Here's how the part is built. I have some questions about the finished solid (model axes, mm). Face numbers are marked on the shaded views. A direction names the side the tool comes from. Round coordinates to 2 decimals unless told otherwise and drop trailing zeros. Order: outer loops, then holes, each group sorted by start corner. A loop starts at its lowest first (then second) coordinate and runs counter-clockwise, first axis right, second up.
```python
from build123d import *

# Parameters (mm, degrees)
SKETCH2_W             = 5.91625
SKETCH2_H             = 9
BOSS_EXTRUDE1_DEPTH   = 2
SKETCH2_W_2           = 9.732
SKETCH2_H_2           = 9.5
BOSS_EXTRUDE1_2_DEPTH = 2
BOSS_EXTRUDE1_3_DEPTH = 2
SKETCH3_W             = 2
SKETCH3_H             = 1
BOSS_EXTRUDE2_DEPTH   = 13
FILLET1_R             = 4
CUT_EXTRUDE1_DEPTH    = 83.031058661
M3_CLEARANCE_HOLE2_D  = 3.6


with BuildPart() as part:
    # Sketch2 → Boss-Extrude1 (new body)
    with BuildSketch(Plane.XY.offset(11.211435671)):
        with Locations((2.267401673, -43.012787822)):
            Rectangle(SKETCH2_W, SKETCH2_H)
    extrude(amount=BOSS_EXTRUDE1_DEPTH)



with BuildPart() as body_2:
    # Sketch2 → Boss-Extrude1 2 (new body)
    with BuildSketch(Plane.XY.offset(11.211435671)):
        with Locations((0.359526673, -72.762787822)):
            Rectangle(SKETCH2_W_2, SKETCH2_H_2)
    extrude(amount=BOSS_EXTRUDE1_2_DEPTH)


with BuildPart() as body_3:
    # Sketch2 → Boss-Extrude1 3 (new body)
    with BuildSketch(Plane.XY.offset(11.211435671)):
        with Locations((0.359526673, -13.262787822)):
            Rectangle(SKETCH2_W_2, SKETCH2_H_2)
    extrude(amount=BOSS_EXTRUDE1_3_DEPTH)


with BuildPart() as part_1:
    add(part.part)

    add(body_2.part)  # Boss-Extrude2 merges body 2

    add(body_3.part)  # Boss-Extrude2 merges body 3
    # Sketch3 → Boss-Extrude2 (add)
    with BuildSketch(Plane.XY.offset(13.211435671)):
        Polygon((-0.690723327, -17.012787822), (-0.690723327, -38.512787822), (-0.690723327, -47.512787822), (-0.690723327, -68.012787822), (1.309276673, -68.012787822), (1.309276673, -17.012787822), align=None)
        with Locations((0.309276673, -68.512787822)):
            Rectangle(SKETCH3_W, SKETCH3_H)
    extrude(amount=BOSS_EXTRUDE2_DEPTH)

    # Fillet1
    # the kernel refuses this fillet: 4 mm, written as the material it adds along each edge
    with BuildSketch(Plane(origin=(-0.690723327, -17.012787822, 13.211435671), x_dir=(0, 0, 1), z_dir=(0, -1, 0)), Plane(origin=(-0.690723327, -68.012787822, 13.211435671), x_dir=(0, 0, 1), z_dir=(0, -1, 0))) as fillet1_piece_1:
        with BuildLine():
            CenterArc((3.995754239, 4), FILLET1_R, 182.64012102, 87.35987898)
            Line((0, 3.81575), (0, 0))
            Line((0, 0), (3.995754239, 0))
        make_face()
    extrude(amount=1)
    with BuildSketch(Plane(origin=(1.309276673, -17.012787822, 13.211435671), x_dir=(0, 1, 0), z_dir=(-1, 0, 0))) as fillet1_piece_2:
        with BuildLine():
            CenterArc((FILLET1_R, -FILLET1_R), FILLET1_R, 90, 90)
            Line((0, -FILLET1_R), (0, 0))
            Line((0, 0), (FILLET1_R, 0))
        make_face()
    extrude(amount=2)
    with BuildSketch(Plane(origin=(1.309276673, -17.012787822, 13.211435671), x_dir=(1, 0, 0), z_dir=(0, -1, 0))) as fillet1_piece_3_section:
        with BuildLine():
            CenterArc((FILLET1_R, FILLET1_R), FILLET1_R, 180, 90)
            Line((0, FILLET1_R), (0, 0))
            Line((0, 0), (FILLET1_R, 0))
        make_face()
    fillet1_piece_3 = extrude(amount=1, mode=Mode.PRIVATE)
    fillet1_piece_3 = split(fillet1_piece_3, bisect_by=Plane(origin=(5.225526673, -17.012787822, 13.211435671), z_dir=(-1, 0, 0)), keep=Keep.TOP, mode=Mode.PRIVATE)
    add(fillet1_piece_3)
    with BuildSketch(Plane(origin=(1.309276673, -38.512787822, 13.211435671), x_dir=(1, 0, 0), z_dir=(0, -1, 0))) as fillet1_piece_4_section:
        with BuildLine():
            CenterArc((FILLET1_R, FILLET1_R), FILLET1_R, 180, 90)
            Line((0, FILLET1_R), (0, 0))
            Line((0, 0), (FILLET1_R, 0))
        make_face()
    fillet1_piece_4 = extrude(amount=9, mode=Mode.PRIVATE)
    fillet1_piece_4 = split(fillet1_piece_4, bisect_by=Plane(origin=(5.225526673, -38.512787822, 13.211435671), z_dir=(-1, 0, 0)), keep=Keep.TOP, mode=Mode.PRIVATE)
    add(fillet1_piece_4)
    with BuildSketch(Plane(origin=(1.309276673, -68.012787822, 13.211435671), x_dir=(1, 0, 0), z_dir=(0, -1, 0))) as fillet1_piece_5_section:
        with BuildLine():
            CenterArc((FILLET1_R, FILLET1_R), FILLET1_R, 180, 90)
            Line((0, FILLET1_R), (0, 0))
            Line((0, 0), (FILLET1_R, 0))
        make_face()
    fillet1_piece_5 = extrude(amount=1, mode=Mode.PRIVATE)
    fillet1_piece_5 = split(fillet1_piece_5, bisect_by=Plane(origin=(5.225526673, -68.012787822, 13.211435671), z_dir=(-1, 0, 0)), keep=Keep.TOP, mode=Mode.PRIVATE)
    add(fillet1_piece_5)
    with BuildSketch(Plane(origin=(-0.690723327, -69.012787822, 13.211435671), x_dir=(0, 0, 1), z_dir=(1, 0, 0))) as fillet1_piece_6:
        with BuildLine():
            CenterArc((FILLET1_R, FILLET1_R), FILLET1_R, 180, 90)
            Line((0, FILLET1_R), (0, 0))
            Line((0, 0), (FILLET1_R, 0))
        make_face()
    extrude(amount=2)
    with BuildSketch(Plane(origin=(-0.690723327, -7.023402225, 13.211435671), x_dir=(0, 0, 1), z_dir=(0, -1, 0))) as fillet1_piece_7a_section:
        with BuildLine():
            CenterArc((3.995754239, 4), FILLET1_R, 182.64012102, 87.35987898)
            Line((0, 3.81575), (0, 0))
            Line((0, 0), (3.995754239, 0))
        make_face()
    fillet1_piece_7a = extrude(amount=10.989385597, mode=Mode.PRIVATE)
    fillet1_piece_7a = split(fillet1_piece_7a, bisect_by=Plane(origin=(-0.690723327, -17.012787822, 13.211435671), z_dir=(0, 1, 0)), keep=Keep.TOP, mode=Mode.PRIVATE)
    fillet1_piece_7a = split(fillet1_piece_7a, bisect_by=Plane(origin=(-0.690723327, -8.512787822, 13.211435671), z_dir=(0, -1, 0)), keep=Keep.TOP, mode=Mode.PRIVATE)
    with BuildSketch(Plane(origin=(1.309276673, -17.012787822, 13.211435671), x_dir=(0, 1, 0), z_dir=(-1, 0, 0))) as fillet1_piece_7b_section:
        with BuildLine():
            CenterArc((FILLET1_R, -FILLET1_R), FILLET1_R, 90, 90)
            Line((0, -FILLET1_R), (0, 0))
            Line((0, 0), (FILLET1_R, 0))
        make_face()
    fillet1_piece_7b = extrude(amount=12, mode=Mode.PRIVATE)
    fillet1_piece_7b = split(fillet1_piece_7b, bisect_by=Plane(origin=(-0.690723327, -17.012787822, 13.211435671), z_dir=(-1, 0, 0)), keep=Keep.TOP, mode=Mode.PRIVATE)
    fillet1_piece_7b = split(fillet1_piece_7b, bisect_by=Plane(origin=(-4.506473327, -17.012787822, 13.211435671), z_dir=(1, 0, 0)), keep=Keep.TOP, mode=Mode.PRIVATE)
    fillet1_piece_7 = fillet1_piece_7a & fillet1_piece_7b
    add(fillet1_piece_7)
    with BuildSketch(Plane(origin=(1.309276673, -7.012787822, 13.211435671), x_dir=(1, 0, 0), z_dir=(0, -1, 0))) as fillet1_piece_8a_section:
        with BuildLine():
            CenterArc((FILLET1_R, FILLET1_R), FILLET1_R, 180, 90)
            Line((0, FILLET1_R), (0, 0))
            Line((0, 0), (FILLET1_R, 0))
        make_face()
    fillet1_piece_8a = extrude(amount=11, mode=Mode.PRIVATE)
    fillet1_piece_8a = split(fillet1_piece_8a, bisect_by=Plane(origin=(1.309276673, -17.012787822, 13.211435671), z_dir=(0, 1, 0)), keep=Keep.TOP, mode=Mode.PRIVATE)
    fillet1_piece_8a = split(fillet1_piece_8a, bisect_by=Plane(origin=(1.309276673, -8.512787822, 13.211435671), z_dir=(0, -1, 0)), keep=Keep.TOP, mode=Mode.PRIVATE)
    with BuildSketch(Plane(origin=(11.309276673, -17.012787822, 13.211435671), x_dir=(0, 1, 0), z_dir=(-1, 0, 0))) as fillet1_piece_8b_section:
        with BuildLine():
            CenterArc((FILLET1_R, -FILLET1_R), FILLET1_R, 90, 90)
            Line((0, -FILLET1_R), (0, 0))
            Line((0, 0), (FILLET1_R, 0))
        make_face()
    fillet1_piece_8b = extrude(amount=12, mode=Mode.PRIVATE)
    fillet1_piece_8b = split(fillet1_piece_8b, bisect_by=Plane(origin=(1.309276673, -17.012787822, 13.211435671), z_dir=(1, 0, 0)), keep=Keep.TOP, mode=Mode.PRIVATE)
    fillet1_piece_8b = split(fillet1_piece_8b, bisect_by=Plane(origin=(5.225526673, -17.012787822, 13.211435671), z_dir=(-1, 0, 0)), keep=Keep.TOP, mode=Mode.PRIVATE)
    fillet1_piece_8 = fillet1_piece_8a & fillet1_piece_8b
    add(fillet1_piece_8)
    with BuildSketch(Plane(origin=(-0.690723327, -68.012787822, 13.211435671), x_dir=(0, 0, 1), z_dir=(0, -1, 0))) as fillet1_piece_9a_section:
        with BuildLine():
            CenterArc((3.995754239, 4), FILLET1_R, 182.64012102, 87.35987898)
            Line((0, 3.81575), (0, 0))
            Line((0, 0), (3.995754239, 0))
        make_face()
    fillet1_piece_9a = extrude(amount=10.989385597, mode=Mode.PRIVATE)
    fillet1_piece_9a = split(fillet1_piece_9a, bisect_by=Plane(origin=(-0.690723327, -69.012787822, 13.211435671), z_dir=(0, -1, 0)), keep=Keep.TOP, mode=Mode.PRIVATE)
    fillet1_piece_9a = split(fillet1_piece_9a, bisect_by=Plane(origin=(-0.690723327, -77.512787822, 13.211435671), z_dir=(0, 1, 0)), keep=Keep.TOP, mode=Mode.PRIVATE)
    with BuildSketch(Plane(origin=(-10.690723327, -69.012787822, 13.211435671), x_dir=(0, 0, 1), z_dir=(1, 0, 0))) as fillet1_piece_9b_section:
        with BuildLine():
            CenterArc((FILLET1_R, FILLET1_R), FILLET1_R, 180, 90)
            Line((0, FILLET1_R), (0, 0))
            Line((0, 0), (FILLET1_R, 0))
        make_face()
    fillet1_piece_9b = extrude(amount=12, mode=Mode.PRIVATE)
    fillet1_piece_9b = split(fillet1_piece_9b, bisect_by=Plane(origin=(-0.690723327, -69.012787822, 13.211435671), z_dir=(-1, 0, 0)), keep=Keep.TOP, mode=Mode.PRIVATE)
    fillet1_piece_9b = split(fillet1_piece_9b, bisect_by=Plane(origin=(-4.506473327, -69.012787822, 13.211435671), z_dir=(1, 0, 0)), keep=Keep.TOP, mode=Mode.PRIVATE)
    fillet1_piece_9 = fillet1_piece_9a & fillet1_piece_9b
    add(fillet1_piece_9)
    with BuildSketch(Plane(origin=(-0.690723327, -69.012787822, 13.211435671), x_dir=(0, 0, 1), z_dir=(1, 0, 0))) as fillet1_piece_10a_section:
        with BuildLine():
            CenterArc((FILLET1_R, FILLET1_R), FILLET1_R, 180, 90)
            Line((0, FILLET1_R), (0, 0))
            Line((0, 0), (FILLET1_R, 0))
        make_face()
    fillet1_piece_10a = extrude(amount=12, mode=Mode.PRIVATE)
    fillet1_piece_10a = split(fillet1_piece_10a, bisect_by=Plane(origin=(1.309276673, -69.012787822, 13.211435671), z_dir=(1, 0, 0)), keep=Keep.TOP, mode=Mode.PRIVATE)
    fillet1_piece_10a = split(fillet1_piece_10a, bisect_by=Plane(origin=(5.225526673, -69.012787822, 13.211435671), z_dir=(-1, 0, 0)), keep=Keep.TOP, mode=Mode.PRIVATE)
    with BuildSketch(Plane(origin=(1.309276673, -68.012787822, 13.211435671), x_dir=(1, 0, 0), z_dir=(0, -1, 0))) as fillet1_piece_10b_section:
        with BuildLine():
            CenterArc((FILLET1_R, FILLET1_R), FILLET1_R, 180, 90)
            Line((0, FILLET1_R), (0, 0))
            Line((0, 0), (FILLET1_R, 0))
        make_face()
    fillet1_piece_10b = extrude(amount=11, mode=Mode.PRIVATE)
    fillet1_piece_10b = split(fillet1_piece_10b, bisect_by=Plane(origin=(1.309276673, -69.012787822, 13.211435671), z_dir=(0, -1, 0)), keep=Keep.TOP, mode=Mode.PRIVATE)
    fillet1_piece_10b = split(fillet1_piece_10b, bisect_by=Plane(origin=(1.309276673, -77.512787822, 13.211435671), z_dir=(0, 1, 0)), keep=Keep.TOP, mode=Mode.PRIVATE)
    fillet1_piece_10 = fillet1_piece_10a & fillet1_piece_10b
    add(fillet1_piece_10)

    # Sketch6 → Cut-Extrude1 (cut, through all)
    with BuildSketch(Plane(origin=(1.309276673, 0, 0), x_dir=(0, 0, -1), z_dir=(1, 0, 0))):
        Polygon((-13.211435671, -18.012787822), (-17.991089167, -28.262787822), (-13.211435671, -38.512787822), align=None)
        Polygon((-17.991089167, -57.762787822), (-13.211435671, -47.512787822), (-13.211435671, -68.012787822), align=None)
    extrude(amount=-CUT_EXTRUDE1_DEPTH, mode=Mode.SUBTRACT)

    # M3 Clearance Hole2 (through all)
    with Locations(Plane(origin=(1.309276673, 0, 0), x_dir=(0, 0, -1), z_dir=(1, 0, 0))):
        with Locations((-22.101262419, -28.262787822), (-22.101262419, -57.762787822)):
            Hole(M3_CLEARANCE_HOLE2_D / 2)


solid = part_1.part
```
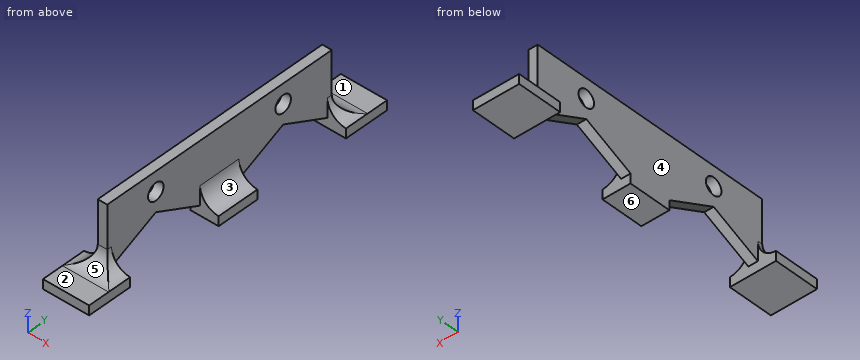
1. If we mould it in two halves opening along Y, with no side actions, what happens to the marked faces 4, 5 and 6? For each: released by +Y, released by -Y, zero draft, split by the parting line, or undercut.
Evaluation:
face 4: undercut
face 5: released by -Y
face 6: zero draft
2. If we section it at C-C, the plane x = -2.5: Write out the boundary of the cut face in (y, z).
Evaluation:
outline: (-77.51, 11.21) - (-68.01, 11.21) - (-68.01, 13.86) - (-70.83, 13.86) arc R4 cw to (-73.01, 13.21) - (-77.51, 13.21) - close; (-18.01, 11.21) - (-8.51, 11.21) - (-8.51, 13.21) - (-13.01, 13.21) arc R4 cw to (-15.2, 13.86) - (-18.01, 13.86) - close
3. I'm going to push flat-ended pins straight in: P1, Ø5, axis at x = 0, y = -37.5, coming from the -Z side; P2, Ø5, axis at y = -67, z = 17.5, coming from the +X side; P3, Ø2, axis at x = 0, z = 20, coming from the +Y side; P4, Ø3, axis at x = 2.5, z = 15, coming from the +Y side. Where does each tip first touch, or does it pass through?
Evaluation:
P1: stops at z = 11.21
P2: stops at x = 1.84
P3: stops at y = -17.01
P4: stops at y = -14.5
4. On a 3-axis mill with a long thin cutter (end or side, diameter ignored), from which of +Z, -Z, +X, -X, +Y, -Y can I reach the whole of each face in a straight line? I mean the marked faces 1, 2 and 3. Say none if no direction works.
Evaluation:
face 1: +Z, +X, -X, +Y
face 2: +Z, +X, -X, -Y
face 3: +Z, +X, +Y, -Y
5. If we section it at A-A, the plane x = 0: Write out the boundary of the cut face in (y, z).
Evaluation:
outline: (-77.51, 11.21) - (-68.01, 11.21) - (-68.01, 13.21) - (-57.76, 17.99) - (-47.51, 13.21) - (-47.51, 11.21) - (-38.51, 11.21) - (-38.51, 13.21) - (-28.26, 17.99) - (-18.01, 13.21) - (-18.01, 11.21) - (-8.51, 11.21) - (-8.51, 13.21) - (-13.01, 13.21) arc R4 cw to (-17.01, 17.21) - (-17.01, 26.21) - (-69.01, 26.21) - (-69.01, 17.21) arc R4 cw to (-73.01, 13.21) - (-77.51, 13.21) - close; hole circle Ø3.6 at (-57.76, 22.1); hole circle Ø3.6 at (-28.26, 22.1)
6. I need wall thicknesses on probe 1 along Y at (x, z) = (-0.5, 12.25); probe 2 along Y at (x, z) = (0.5, 17.25); probe 3 along Y at (x, z) = (-0.75, 15.5). Which ranges of each line are inside material? Lowest first, please.
Evaluation:
probe 1: y = -77.51 to -68.01, -47.51 to -38.51, -18.01 to -8.51
probe 2: y = -69.01 to -59.35, -56.17 to -29.85, -26.67 to -17.01
probe 3: y = -69.4 to -68.01, -18.01 to -16.63
7. If we section it at B-B, the plane z = 22.5: Write out the boundary of the cut face in (x, y), and give its area (3 significant figures).
Evaluation:
outline: (-0.69, -69.01) - (1.31, -69.01) - (1.31, -59.52) - (-0.69, -59.52) - close; (-0.69, -56.01) - (1.31, -56.01) - (1.31, -30.02) - (-0.69, -30.02) - close; (-0.69, -26.51) - (1.31, -26.51) - (1.31, -17.01) - (-0.69, -17.01) - close
area: 90.0 mm2
8. If we section it at D-D, the plane y = -72: Write out the boundary of the cut face in (x, z), and give its area (3 significant figures).
Evaluation:
outline: (-4.51, 11.21) - (5.23, 11.21) - (5.23, 13.21) arc R4 cw to (4.3, 13.34) - (-3.66, 13.34) arc R4 cw to (-4.51, 13.21) - close
area: 20.6 mm2
